from build123d import *

# Parameters (mm, degrees)
SKETCH_1_R          = 18.5
SKETCH_1_R_2        = 1.5
EXTRUDE_1_DEPTH     = 23
SKETCH_1_3_R        = 6
SKETCH_1_3_R_2      = 3
EXTRUDE_2_DEPTH     = 6
SKETCH_1_4_R        = 3
EXTRUDE_3_DEPTH     = 18
SKETCH_1_5_R        = 16.5
SKETCH_1_5_R_2      = 1.5
SKETCH_1_5_R_3      = 6
SKETCH_1_5_R_4      = 3
EXTRUDE_5_DEPTH     = 53
SKETCH_1_6_R        = 1.5
CUT_EXTRUDE_3_DEPTH = 10


with BuildPart() as part:
    # Sketch 1 → Extrude 1 (new body)
    with BuildSketch(Plane.XY):
        Circle(SKETCH_1_R)
        with Locations((-15.5, 0)):
            Circle(SKETCH_1_R_2, mode=Mode.SUBTRACT)
        with Locations((-7.75, 13.423393759)):
            Circle(SKETCH_1_R_2, mode=Mode.SUBTRACT)
        with Locations((7.75, 13.423393759)):
            Circle(SKETCH_1_R_2, mode=Mode.SUBTRACT)
        with Locations((15.5, 0)):
            Circle(SKETCH_1_R_2, mode=Mode.SUBTRACT)
        with Locations((7.75, -13.423393759)):
            Circle(SKETCH_1_R_2, mode=Mode.SUBTRACT)
        with Locations((-7.75, -13.423393759)):
            Circle(SKETCH_1_R_2, mode=Mode.SUBTRACT)
    extrude(amount=EXTRUDE_1_DEPTH)

    # Sketch 1_3 → Extrude 2 (add)
    with BuildSketch(Plane.XY):
        with Locations((0, 7)):
            Circle(SKETCH_1_3_R)
        with Locations((0, 7)):
            Circle(SKETCH_1_3_R_2, mode=Mode.SUBTRACT)
    extrude(amount=-EXTRUDE_2_DEPTH)

    # Sketch 1_4 → Extrude 3 (add)
    with BuildSketch(Plane.XY):
        with Locations((0, 7)):
            Circle(SKETCH_1_4_R)
    extrude(amount=-EXTRUDE_3_DEPTH)

    # Sketch 1_5 → Extrude 5 (add)
    with BuildSketch(Plane.XY):
        Circle(SKETCH_1_5_R)
        with Locations((-7.75, 13.423393759)):
            Circle(SKETCH_1_5_R_2)
        with Locations((-15.5, 0)):
            Circle(SKETCH_1_5_R_2)
        with Locations((-7.75, -13.423393759)):
            Circle(SKETCH_1_5_R_2)
        with Locations((7.75, -13.423393759)):
            Circle(SKETCH_1_5_R_2)
        with Locations((7.75, 13.423393759)):
            Circle(SKETCH_1_5_R_2)
        with Locations((15.5, 0)):
            Circle(SKETCH_1_5_R_2)
        Circle(SKETCH_1_5_R)
        with Locations((0, 7)):
            Circle(SKETCH_1_5_R_3, mode=Mode.SUBTRACT)
        with Locations((0, 7)):
            Circle(SKETCH_1_5_R_3)
        with Locations((0, 7)):
            Circle(SKETCH_1_5_R_4, mode=Mode.SUBTRACT)
        with Locations((0, 7)):
            Circle(SKETCH_1_5_R_4)
    extrude(amount=EXTRUDE_5_DEPTH)

    # Sketch 1_6 → Cut-Extrude 3 (cut)
    with BuildSketch(Plane.XY):
        with Locations((-15.5, 0)):
            Circle(SKETCH_1_6_R)
        with Locations((-7.75, 13.423393759)):
            Circle(SKETCH_1_6_R)
        with Locations((7.75, 13.423393759)):
            Circle(SKETCH_1_6_R)
        with Locations((15.5, 0)):
            Circle(SKETCH_1_6_R)
        with Locations((7.75, -13.423393759)):
            Circle(SKETCH_1_6_R)
        with Locations((-7.75, -13.423393759)):
            Circle(SKETCH_1_6_R)
    extrude(amount=CUT_EXTRUDE_3_DEPTH, mode=Mode.SUBTRACT)


solid = part.part
Geometry: final body of the model. Coordinates: model frame, mm. A direction names the side the tool comes from. Give positions to 0.01 mm unless a question says otherwise; leave off trailing zeros. Loops run counter-clockwise (first coordinate to the right, second up) from the corner with the lowest first, then second, coordinate; pieces in that order, holes last. Notation, with made-up numbers: (-35.5, 72) - (-30.5, 72) arc R28 ccw to (-30.5, 91) - close; hole circle Ø5 at (59, -2). An arc over 180 degrees is marked (long way). One line per question, with ' | ' between items. Start each with the question number.
(1) Section query B-B on y = 0. Return loops of the section in (x, z), then the cut area to 3 significant figures.
(2) Ray query, line 1 (Y direction, x = 7.75, z = 8); line 2 (Z direction, x = 7, y = 11.5); line 3 (Y direction, x = 16, z = 8.5). Return the intervals inside material, ascending. Write a range as from..to.
(3) Section query A-A on z = 43. Return loops of the section in (x, y), then the cut area to 3 significant figures.
(4) Contact query for flat-ended pins moving along their axis: pin 1 (8 mm diameter, centred on y = -14, z = 30.5, fed in from -X); pin 2 (18.5 mm diameter, centred on x = 0, y = -8, fed in from -Z); pin 3 (12 mm diameter, centred on x = 7.5, z = 43.5, fed in from -Y). Output: stop coordinate, or through.
(5) Pull-direction query (Y, two-part tool) for faces 1 (the cylindrical face through (-14.237, 8.341, 37.79)), 2 (the cylindrical face through (-8.08, 11.96, 4.93)), 3 (the cylindrical face through (-3, 7, -12)); classes: released by +Y, released by -Y, zero draft, split by the parting line, or undercut.
(6) Section query D-D on x = -15.5. Return loops of the section in (y, z), then the cut area to 3 significant figures.
(7) Reachability of faces 4 (the cylindrical face through (14.34, 8.16, 37.79)), 5 (the cylindrical face through (-14.34, -8.16, 37.79)), 6 (the flat face through (15, 0, 10)), 7 (the cylindrical face through (-17, 0, 38)) from +Z, -Z, +X, -X, +Y, -Y: full face, straight path, thin tool, end or side. Return the list, or none.
(8) Section query C-C on x = 0. Return loops of the section in (y, z).
The answers:
1) outline: (-18.5, 0) - (-17, 0) - (-17, 10) - (-14, 10) - (-14, 0) - (14, 0) - (14, 10) - (17, 10) - (17, 0) - (18.5, 0) - (18.5, 23) - (17, 23) - (17, 53) - (-17, 53) - (-17, 23) - (-18.5, 23) - close | area: 1,810 mm2
2) line 1: -16.8..-14.92, -11.92..11.92, 14.92..16.8 | line 2: 0..53 | line 3: -9.29..-1.41, 1.41..9.29
3) outline: (-16.46, -1.15) arc R16.5 ccw to (-9.23, -13.68) arc R1.5 ccw to (-7.23, -14.83) arc R16.5 ccw to (7.23, -14.83) arc R1.5 ccw to (9.23, -13.68) arc R16.5 ccw to (16.46, -1.15) arc R1.5 ccw to (16.46, 1.15) arc R16.5 ccw to (9.23, 13.68) arc R1.5 ccw to (7.23, 14.83) arc R16.5 ccw to (-7.23, 14.83) arc R1.5 ccw to (-9.23, 13.68) arc R16.5 ccw to (-16.46, 1.15) arc R1.5 ccw to start | area: 860 mm2
4) pin 1: x = -13.12 | pin 2: z = -6 | pin 3: y = -16.43
5) face 1: released by +Y | face 2: undercut | face 3: split by the parting line
6) outline: (-10.1, 0) - (-1.5, 0) - (-1.5, 10) - (1.5, 10) - (1.5, 0) - (10.1, 0) - (10.1, 23) - (5.66, 23) - (5.66, 53) - (-5.66, 53) - (-5.66, 23) - (-10.1, 23) - close | area: 774 mm2
7) face 4: +Z, +X, +Y | face 5: +Z, -X, -Y | face 6: -Z | face 7: +Z, -X
8) outline: (-18.5, 0) - (1, 0) - (1, -6) - (4, -6) - (4, -18) - (10, -18) - (10, -6) - (13, -6) - (13, 0) - (18.5, 0) - (18.5, 23) - (16.5, 23) - (16.5, 53) - (-16.5, 53) - (-16.5, 23) - (-18.5, 23) - close
